Geometry: final body of the model. Coordinates: model frame, mm. Face numbers are marked on the shaded views. Give positions to 0.01 mm unless a question says otherwise; leave off trailing zeros. Loops run counter-clockwise (first coordinate to the right, second up) from the corner with the lowest first, then second, coordinate; pieces in that order, holes last.
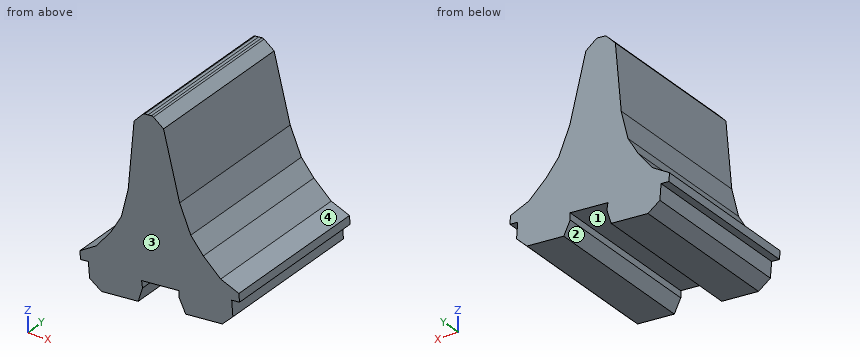
from build123d import *

# Parameters (mm, degrees)
F1_DEPTH = 34


with BuildPart() as f1:
    # F0 (on Front) → F1 (new body)
    with BuildSketch(Plane.XZ):
        with BuildLine():
            Line((-12.198149, -14.302597), (-12.427167, -12.850712))
            Line((-12.427167, -12.850712), (-4.222136, -12.207562))
            Line((-4.222136, -12.207562), (-4.222136, -13.677399))
            Line((-4.222136, -13.677399), (-2.822079, -16.533816))
            Line((-2.822079, -16.533816), (5.16684, -15.907606))
            Line((5.16684, -15.907606), (7.443612, -13.677399))
            Line((7.443612, -13.677399), (7.182818, -10.35031))
            Line((7.182818, -10.35031), (8.885174, -10.216871))
            Line((8.885174, -10.216871), (8.748127, -8.468476))
            Line((8.748127, -8.468476), (4.78861, -6.830055))
            Line((4.78861, -6.830055), (1.006297, -3.350328))
            Line((1.006297, -3.350328), (-1.716968, 0))
            Line((-1.716968, 0), (-4.137649, 5.802869))
            Line((-4.137649, 5.802869), (-7.634035, 19.805321))
            Line((-7.634035, 19.805321), (-9.829951, 21.48903))
            ThreePointArc((-9.829951, 21.48903), (-10.036781, 21.594364), (-10.267614, 21.618659))
            Line((-10.267614, 21.618659), (-10.99684, 21.561499))
            Line((-10.99684, 21.561499), (-11.726065, 21.504339))
            Line((-11.726065, 21.504339), (-12.138186, 21.308099))
            Line((-12.138186, 21.308099), (-14.04494, 19.302804))
            Line((-14.04494, 19.302804), (-15.316869, 4.926588))
            Line((-15.316869, 4.926588), (-16.803827, -1.182581))
            Line((-16.803827, -1.182581), (-18.97181, -4.916308))
            Line((-18.97181, -4.916308), (-22.165744, -8.942867))
            Line((-22.165744, -8.942867), (-25.821616, -11.178218))
            Line((-25.821616, -11.178218), (-25.684568, -12.926614))
            Line((-25.684568, -12.926614), (-23.982212, -12.793175))
            Line((-23.982212, -12.793175), (-23.721419, -16.120264))
            Line((-23.721419, -16.120264), (-21.124961, -17.968484))
            Line((-21.124961, -17.968484), (-13.136041, -17.342274))
            Line((-13.136041, -17.342274), (-12.198149, -14.302597))
        make_face()
    extrude(amount=F1_DEPTH)


solid = f1.part
Item 1: Section query C-C on x = 2.5. Return loops of the section in (y, z), plus the area to 3 significant figures.
Values follow:
outline: (-34, -16.12) - (0, -16.12) - (0, -4.72) - (-34, -4.72) - close
area: 387 mm2
Item 2: Pin query (flat end, axial travel): pin 1 (3 mm diameter, centred on x = -7.5, y = -3.5, fed in from +Z); pin 2 (1 mm diameter, centred on y = -15.5, z = 16.5, fed in from +X); pin 3 (4 mm diameter, centred on y = -3.5, z = -1, fed in from -X). Return the tip coordinate at first contact, or that it passes through.
Values follow:
pin 1: stops at z = 20.85
pin 2: stops at x = -6.68
pin 3: stops at x = -17.86
Item 3: Draft query along X for the marked faces 1, 2, 3 and 4. Return one class per face: +X half, -X half, draft (parallel to the pull), parting line (faces both ways), or undercut.
Values follow:
face 1: undercut
face 2: undercut
face 3: draft
face 4: +X half
Item 4: Section query B-B on z = 11. Return loops of the section in (x, y).
Values follow:
outline: (-14.78, -34) - (-5.44, -34) - (-5.44, 0) - (-14.78, 0) - close
Item 5: Ray query, probe 1 along X at (y, z) = (-4, -13.5); probe 2 along Z at (x, y) = (3.5, -14); probe 3 along X at (y, z) = (-20.5, -10). Return the intervals inside material, ascending.
Values follow:
probe 1: x = -23.93 to -12.32, -4.22 to 7.43
probe 2: z = -16.04 to -5.64
probe 3: x = -23.89 to 8.87
